Build history of the part. All positions in model axes, mm. Coordinates: 2 decimals unless noted, no trailing zeros. Loops run counter-clockwise (first coordinate to the right, second up) from the corner with the lowest first, then second, coordinate; pieces in that order, holes last.
Item 1: Mould opens along X. For faces 1 (the face through (-0.34, -1.55, 0.05)), 2 (the face through (-1, -1, -3.175)), 3 (the face through (0.757, 0.238, -1.998)), 4 (the face through (-0.69, -3.1, -1.57)) say: released by +X, released by -X, zero draft, split by the parting line, or undercut.
Item 2: Flat gauge pins, fed straight in: pin 1 (1.9 mm diameter, centred on x = 0, y = 0, fed in from +Z); pin 2 (2 mm diameter, centred on y = -1.5, z = 0, fed in from -X); pin 3 (2.5 mm diameter, centred on x = 0, y = 0, fed in from +Z). Where does each tip first touch, or does it go through?
Item 3: Drill centre lines: line 1 along Z through (x, y) = (-2, -2) (3 decimals); line 2 along Y through (x, z) = (0, -2) (3 decimals); line 3 along X through (y, z) = (0, 4.4). Where is each one in solid material? Low to high.
Item 4: Cut at C-C (x = 1). List the corners of the cut face in (y, z) (3 decimals), and give its area (3 significant figures).
Item 5: Cut at B-B (z = 1.25). List the corners of the cut face in (x, y).
from build123d import *

# Parameters (mm, degrees)
F3_DEPTH      = 3.176
F3_DEPTH_BACK = 25.4


with BuildPart() as f1:
    # F0 (on Front) → F1 (revolve)
    with BuildSketch(Plane.XZ):
        with BuildLine():
            Line((1.5875, 0.5691135997), (1.5875, 0))
            Line((1.5875, 0), (2.2033676498, 0))
            ThreePointArc((2.2033676498, 0), (3.1515176365, 2.6714368781), (1.5875, 5.035630657))
            Line((1.5875, 5.035630657), (1.5875, 4.0028864003))
            ThreePointArc((1.5875, 4.0028864003), (2.3383445344, 2.286), (1.5875, 0.5691135997))
        make_face()
        with BuildLine():
            ThreePointArc((1.5875, -0.463630657), (1.2016326584, -0.6528269691), (0.79375, -0.7881805311))
            Line((0.79375, -0.7881805311), (0.79375, -0.889))
            Line((0.79375, -0.889), (0.79375, -3.175))
            Line((0.79375, -3.175), (3.175, -3.175))
            Line((3.175, -3.175), (3.175, 0))
            Line((3.175, 0), (2.2033676498, 0))
            ThreePointArc((2.2033676498, 0), (1.9095569463, -0.2505758946), (1.5875, -0.463630657))
        make_face()
        with BuildLine():
            Line((2.2033676498, 0), (1.5875, 0))
            Line((1.5875, 0), (1.5875, -0.463630657))
            ThreePointArc((1.5875, -0.463630657), (1.9095569463, -0.2505758946), (2.2033676498, 0))
        make_face()
    revolve(axis=Axis((0, 0, 2.286), (0, 0, 1)))

    # F2 (on Front) → F3 (cut, two sides)
    with BuildSketch(Plane.XZ) as f3_sk:
        with BuildLine():
            ThreePointArc((0, 0.508), (1.2572358569, 1.0287641431), (1.778, 2.286))
            ThreePointArc((1.778, 2.286), (-1.2572358569, 3.5432358569), (0, 0.508))
        make_face()
    extrude(amount=F3_DEPTH, mode=Mode.SUBTRACT)
    extrude(f3_sk.sketch, amount=-F3_DEPTH_BACK, mode=Mode.SUBTRACT)


solid = f1.part
Filled sheet:
1. face 1: undercut
1. face 2: zero draft
1. face 3: undercut
1. face 4: split by the parting line
2. pin 1: stops at z = -0.74
2. pin 2: stops at x = -3.14
2. pin 3: stops at z = -0.63
3. line 1: z = -3.175 to 0, 0.844 to 3.728
3. line 2: y = -3.175 to -0.794, 0.794 to 3.175
3. line 3: x = -2.37 to -1.59, 1.59 to 2.37
4. outline: (-3.013, -3.175) - (3.013, -3.175) - (3.013, 0) - (1.963, 0) arc R3.013 ccw to (2.63, 0.816) - (1.519, 0.816) arc R2.114 cw to (1.233, 0.569) - (1.233, -0.464) arc R3.013 cw to (-1.233, -0.464) - (-1.233, 0.569) arc R2.114 cw to (-1.519, 0.816) - (-2.63, 0.816) arc R3.013 ccw to (-1.963, 0) - (-3.013, 0) - close; (-2.63, 3.756) - (-1.519, 3.756) arc R2.114 cw to (-1.233, 4.003) - (-1.233, 5.036) arc R3.013 ccw to start; (1.233, 4.003) arc R2.114 cw to (1.519, 3.756) - (2.63, 3.756) arc R3.013 ccw to (1.233, 5.036) - close
4. area: 21.4 mm2
5. outline: (-1.44, -2.63) - (-1.44, -1.52) arc R2.1 cw to (-1.44, 1.52) - (-1.44, 2.63) arc R3 ccw to start; (1.44, -2.63) arc R3 ccw to (1.44, 2.63) - (1.44, 1.52) arc R2.1 cw to (1.44, -1.52) - close
